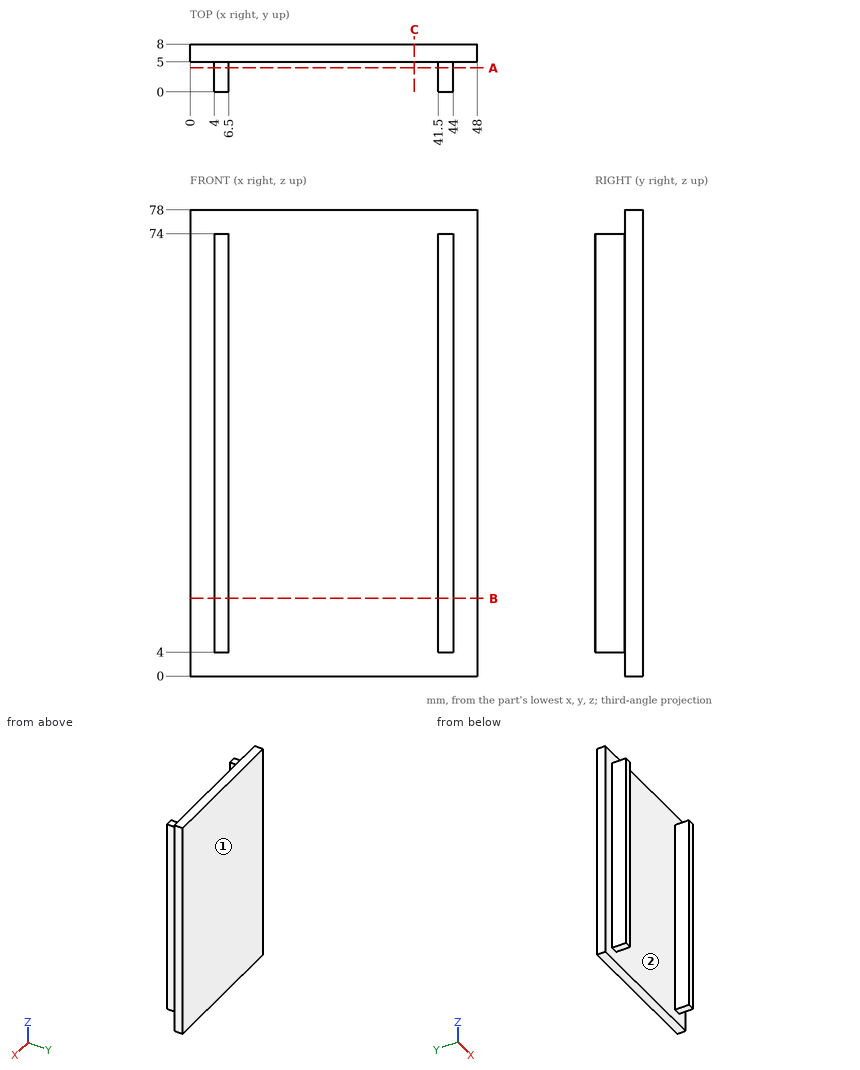
Answer from the drawing. Dimensions are ordinates in mm from the lowest x, y and z of the part. Round coordinates to 2 decimals unless told otherwise and drop trailing zeros. Write each loop counter-clockwise with the first axis right and the second up, starting at its lowest first coordinate (ties: lowest second). Pieces come first, ordered by that corner, then holes.
1. The part is cut by section B-B, the plane z = 13. Determine the outline of the cut face in (x, y), then the cut area to 3 significant figures.
2. Determine the mould class of the marked faces 1 and 2 for opening direction X: pulls with the +X half, pulls with the -X half, needs draft (parallel to the pull), parting line crosses it, or undercut.
3. The part is cut by section C-C, the plane x = 37.5. Determine the outline of the cut face in (y, z).
4. The part is cut by section A-A, the plane y = 4. Determine the outline of the cut face in (x, z), then the cut area to 3 significant figures.
5. Straight lines are drawn through the part: L1, parallel to X at y = 1.25, z = 45.5; L2, parallel to Y at x = 32, z = 53. For each, find the intervals that lie inside material, in ascending order.
6. Given pin 1 Ø1.5 at (y, z) = (2, 26) entering from -X; pin 2 Ø3 at (x, y) = (5.5, 2) entering from -Z; pin 3 Ø2 at (x, z) = (24.5, 63) entering from -Y, each flat-ended and moving along its own axis, determine where each tip first touches the part or whether it passes through.
Values:
1. outline: (0, 5) - (4, 5) - (4, 0) - (6.5, 0) - (6.5, 5) - (41.5, 5) - (41.5, 0) - (44, 0) - (44, 5) - (48, 5) - (48, 8) - (0, 8) - close
1. area: 169 mm2
2. face 1: needs draft
2. face 2: undercut
3. outline: (5, 0) - (8, 0) - (8, 78) - (5, 78) - close
4. outline: (4, 4) - (6.5, 4) - (6.5, 74) - (4, 74) - close; (41.5, 4) - (44, 4) - (44, 74) - (41.5, 74) - close
4. area: 350 mm2
5. L1: x = 4 to 6.5, 41.5 to 44
5. L2: y = 5 to 8
6. pin 1: stops at x = 4
6. pin 2: stops at z = 4
6. pin 3: stops at y = 5
